Geometry: final body of the model. Coordinates: model frame, mm. A direction names the side the tool comes from. Give positions to 0.01 mm unless a question says otherwise; leave off trailing zeros. Write each loop counter-clockwise with the first axis right and the second up, starting at its lowest first coordinate (ties: lowest second). Pieces come first, ordered by that corner, then holes. Notation, with made-up numbers: M 89,11.5 L 130,11.5 A17 cw 130,23.5 Z; hole C 88,17 d1. An arc over 180 degrees is marked long. Answer as a JSON object with one key per item and string values.
from build123d import *

# Parameters (mm, degrees)
F0_W      = 31.75
F0_H      = 9.525
F1_DEPTH  = 3.175
F4_R      = 2.286
F8_R      = 2.286
F11_DEPTH = 3.175
F13_DEPTH = 52.79898
F15_DEPTH = 25.4
F17_DEPTH = 2


with BuildPart() as f1:
    # F0 (on Top) → F1 (new body)
    with BuildSketch(Plane.XY):
        with Locations((15.875, 4.7625)):
            Rectangle(F0_W, F0_H)
    extrude(amount=F1_DEPTH)

    # F5: sweep along a path in F3
    with BuildLine(Plane.YZ.offset(28.575)) as f5_path:
        Line((7.1374, 3.175), (7.1374, 9.525))
        Line((7.1374, 9.525), (11.6275280605, 14.0151280605))
    # F4 (on face) → F5 (sweep)
    with BuildSketch(Plane.XY.offset(3.175)):
        with Locations((28.575, 7.1374)):
            Circle(F4_R)
    sweep(path=f5_path.line, transition=Transition.RIGHT)

    # F9: sweep along a path in F7
    with BuildLine(Plane.YZ.offset(3.175)) as f9_path:
        Line((7.1374, 3.175), (7.1374, 9.525))
        Line((7.1374, 9.525), (11.6275280605, 14.0151280605))
    # F8 (on face) → F9 (sweep)
    with BuildSketch(Plane.XY.offset(3.175)):
        with Locations((3.175, 7.1374)):
            Circle(F8_R)
    sweep(path=f9_path.line, transition=Transition.RIGHT)

    # F10 (on face) → F11 (join, through all)
    with BuildSketch(Plane.XY.offset(3.175)):
        with BuildLine():
            Line((25.3239712887, -6.4260287113), (37.2530060984, 5.5030060984))
            ThreePointArc((37.2530060984, 5.5030060984), (15.875, 13.7786934298), (-5.5030060984, 5.5030060984))
            Line((-5.5030060984, 5.5030060984), (6.4260287113, -6.4260287113))
            ThreePointArc((6.4260287113, -6.4260287113), (15.875, 0), (25.3239712887, -6.4260287113))
        make_face()
    extrude(amount=-F11_DEPTH)

    # F12 (on face) → F13 (join)
    with BuildSketch(Plane(origin=(0, 0, 0), x_dir=(1, 0, 0), z_dir=(0, 0, -1))):
        with BuildLine():
            Line((6.4260287113, 6.4260287113), (4.9077839908, 4.9077839908))
            ThreePointArc((4.9077839908, 4.9077839908), (15.875, -2), (26.8422160092, 4.9077839908))
            Line((26.8422160092, 4.9077839908), (25.3239712887, 6.4260287113))
            ThreePointArc((25.3239712887, 6.4260287113), (15.875, 0), (6.4260287113, 6.4260287113))
        make_face()
    extrude(amount=F13_DEPTH)

    # F14 (on face) → F15 (cut)
    with BuildSketch(Plane(origin=(0, 12.8213280605, 12.8213280605), x_dir=(1, 0, 0), z_dir=(0, 0.7071067812, 0.7071067812))):
        Polygon((3.175, -3.9742881508), (2.4454922036, -3.9742881508), (2.4454922036, -10.2548293379), (29.3045077964, -10.2548293379), (29.3045077964, -3.9742881508), align=None)
    extrude(amount=-F15_DEPTH, mode=Mode.SUBTRACT)

    # F16 (on face) → F17 (join)
    with BuildSketch(Plane(origin=(0, 0, -52.79898), x_dir=(1, 0, 0), z_dir=(0, 0, -1))):
        with BuildLine():
            ThreePointArc((17.4591143082, -1.8963751542), (15.875, -2), (14.2908856918, -1.8963751542))
            ThreePointArc((14.2908856918, -1.8963751542), (15.875, -3.5875), (17.4591143082, -1.8963751542))
        make_face()
    extrude(amount=-F17_DEPTH)


solid = f1.part
1) Cut plane A-A on z = -24. Return loops of the section in (x, y) (3 decimals).
Geometry check:
{"outline": "M 4.908,-4.908 L 6.426,-6.426 A10.16 cw 25.324,-6.426 L 26.842,-4.908 A12.16 ccw Z"}
2) Cut plane C-C on x = 33. Return loops of the section in (y, z) (3 decimals).
Geometry check:
{"outline": "M 1.25,0 L 8.764,0 L 8.764,3.175 L 1.25,3.175 Z"}
3) Line query: line 1 (Z direction, x = 25.5, y = 0) (3 decimals); line 2 (X direction, y = -2.5, z = -19); line 3 (X direction, y = -2, z = -10). Output: solid intervals per line, ascending. Write a range as from..to.
Geometry check:
{"line 1": "z = 0..3.175", "line 2": "x = 6.43..9.2, 22.55..25.32", "line 3": "x = 6.86..9.82, 21.93..24.89"}
4) Cut plane B-B on x = 10.5. Return loops of the section in (y, z) (3 decimals), and give its area (3 significant figures).
Geometry check:
{"outline": "M -1.538,-52.799 L 0.748,-52.799 L 0.748,0 L 13.32,0 L 13.32,3.175 L -1.538,3.175 Z", "area": "168 mm2"}
5) Contact query for flat-ended pins moving along their axis: P1, Ø0.8, axis at x = 15, y = 3, coming from the +Z side (3 decimals); P2, Ø10, axis at y = 3.5, z = -14.5, coming from the -X side; P3, Ø4, axis at x = 1.5, y = 3.5, coming from the +Z side. Output: stop coordinate, or through.
Geometry check:
{"P1": "stops at z = 3.175", "P2": "stops at x = 7.34", "P3": "stops at z = 10.72"}
6) Set-up query: faces 4 (the flat face through (5.9, -3.52, 2.1)), 5 (the cylindrical face through (2.7, 4.9, 6.1)), 6 (the cylindrical face through (16.203, 13.777, 1.61)). Return all of +Z, -Z, +X, -X, +Y, -Y with unobstructed straight access to the full face (end or side cutting, diameter ignored); none if empty.
Geometry check:
{"face 4": "+Z, +X, -X, -Y", "face 5": "none", "face 6": "-Z, +Y"}
7) Pull-direction query (X, two-part tool) for faces 1 (the flat face through (26.46, -5.29, -16.39)), 2 (the flat face through (16, 3, -50.799)), 3 (the flat face through (16, 6, 3.175)); classes: pulls with the +X half, pulls with the -X half, needs draft (parallel to the pull), parting line crosses it, or undercut.
Geometry check:
{"face 1": "pulls with the +X half", "face 2": "needs draft", "face 3": "undercut"}
